from build123d import *

# Parameters (mm, degrees)
F1_W          = 5.870015
F1_H          = 6.290437
F2_DEPTH      = 25
F5_R          = 1.924838
F5_R_2        = 2
F6_DEPTH      = 10
F6_DEPTH_BACK = 10


with BuildPart() as f2:
    # F1 (on Front) → F2 (new body)
    with BuildSketch(Plane.XZ):
        with Locations((-3.029539, -0.13159)):
            Rectangle(F1_W, F1_H)
    extrude(amount=F2_DEPTH)

    # F0 (on Front) → F4 section 0
    with BuildSketch(Plane.XZ):
        with BuildLine():
            ThreePointArc((-15.948061, 4.263329), (-14.5, 0), (-15.948061, -4.263329))
            Line((-15.948061, -4.263329), (12.936951, -6.90465))
            ThreePointArc((12.936951, -6.90465), (10.5, 0), (12.936951, 6.90465))
            Line((12.936951, 6.90465), (-15.948061, 4.263329))
        make_face()
    # F3 (on face) → F4 section 1
    with BuildSketch(Plane.XZ.offset(25)):
        with BuildLine():
            ThreePointArc((-15.948061, 4.263329), (-14.500061, -0.029295), (-15.983939, -4.309649))
            Line((-15.983939, -4.309649), (5.2341, -7.625162))
            ThreePointArc((5.2341, -7.625162), (2.500149, -0.059857), (5.158492, 7.532345))
            Line((5.158492, 7.532345), (-15.948061, 4.263329))
        make_face()
    loft()

    # F5 (on Top) → F6 (cut, two sides)
    with BuildSketch(Plane.XY) as f6_sk:
        with Locations((-10.290117, -19.614996)):
            Circle(F5_R)
        with Locations((0.45808, -19.614996)):
            Circle(F5_R_2)
    extrude(amount=F6_DEPTH, mode=Mode.SUBTRACT)
    extrude(f6_sk.sketch, amount=-F6_DEPTH_BACK, mode=Mode.SUBTRACT)


solid = f2.part
Verification items for the finished model (mm, model axes). Give positions to 0.01 mm unless a question says otherwise; leave off trailing zeros. Write item = value, one per line. Start each with the question number.
Q1. Thickness scan on line 1 (X direction, y = -20.25, z = -2); line 2 (Y direction, x = -0.5, z = -0.5); line 3 (Z direction, x = 8, y = -3.5). Record the ranges inside material, lowest first.
Q2. Depth check by flat-ended pin: P1, Ø4, axis at y = -19, z = -1, coming from the -X side; P2, Ø4, axis at x = -0.5, y = -16, coming from the -Z side; P3, Ø6, axis at x = -10.29, y = -19.61, coming from the +Z side. Enter the tip coordinate at first touch or a pass-through.
Q3. Cross-section at A-A, the plane y = -20.5. State how many separate pieces and enclosed holes the cut face has, and give its area (3 significant figures).
Q4. Mould release check, pull along Y, two halves, no side actions. Record for faces 1 (the face through (1.533, -17.929, -0.127)), 2 (the face through (-4, -25, -1)), 3 (the face through (0, 0, -1)): released by +Y, released by -Y, zero draft, split by the parting line, or undercut.
Answer key:
q1.line_1 = -14.79 to -12.11, -8.47 to -1.44, 2.35 to 4.19
q1.line_2 = -25 to -21.37, -17.86 to 0
q1.line_3 = -6.63 to 6.61
q2.P1 = -15.18
q2.P2 = -6.55
q2.P3 = 5.46
q3.separate_pieces = 3
q3.enclosed_holes = 0
q3.area = 147 mm^2
q4.face_1 = undercut
q4.face_2 = released by -Y
q4.face_3 = released by +Y
